```python
from build123d import *

# Parameters (mm, degrees)
SKETCH1_W           = 105
SKETCH1_H           = 105
BOSS_EXTRUDE1_DEPTH = 5
SKETCH2_R           = 5
CUT_EXTRUDE1_DEPTH  = 5
CUT_EXTRUDE2_DEPTH  = 3
FILLET1_R           = 1


with BuildPart() as part:
    # Sketch1 → Boss-Extrude1 (new body)
    with BuildSketch(Plane(origin=(0, 0, 0), x_dir=(1, 0, 0), z_dir=(0, 1, 0))):
        Rectangle(SKETCH1_W, SKETCH1_H)
    extrude(amount=BOSS_EXTRUDE1_DEPTH)

    # Sketch2 → Cut-Extrude1 (cut)
    with BuildSketch(Plane(origin=(0, 5, 0), x_dir=(1, 0, 0), z_dir=(0, 1, 0))):
        with Locations(Location((0, 0, 0), (0, 0, 270))):
            Circle(SKETCH2_R)
    extrude(amount=-CUT_EXTRUDE1_DEPTH, mode=Mode.SUBTRACT)

    # Sketch3 → Cut-Extrude2 (cut)
    with BuildSketch(Plane(origin=(0, 5, 0), x_dir=(1, 0, 0), z_dir=(0, 1, 0))):
        with BuildLine():
            Line((-49.5, -50), (49.5, -50))
            ThreePointArc((49.5, -50), (49.853553391, -49.853553391), (50, -49.5))
            Line((50, -49.5), (50, 49.5))
            ThreePointArc((50, 49.5), (49.853553391, 49.853553391), (49.5, 50))
            Line((49.5, 50), (-49.5, 50))
            ThreePointArc((-49.5, 50), (-49.853553391, 49.853553391), (-50, 49.5))
            Line((-50, 49.5), (-50, -49.5))
            ThreePointArc((-50, -49.5), (-49.853553391, -49.853553391), (-49.5, -50))
        make_face()
    extrude(amount=-CUT_EXTRUDE2_DEPTH, mode=Mode.SUBTRACT)

    # Fillet1
    fillet1_edges = [part.edges().sort_by_distance(p)[0] for p in [
        (52.5, 2.5, 52.5),
        (-52.5, 2.5, 52.5),
        (-52.5, 2.5, -52.5),
        (52.5, 2.5, -52.5),
    ]]
    fillet(fillet1_edges, radius=FILLET1_R)


solid = part.part
```
Input: part model. Units: mm. Frame: model coordinates. A direction names the side the tool comes from. Give positions to 0.01 mm unless a question says otherwise; leave off trailing zeros. Loops run counter-clockwise (first coordinate to the right, second up) from the corner with the lowest first, then second, coordinate; pieces in that order, holes last. Notation, with made-up numbers: M -39.75,-37 L 8.25,-37 A3 ccw 8.25,-32 Z; hole C 29,9.5 d1. An arc over 180 degrees is marked long. Answer as CSV lines item,"result". Start each with the question number.
1. Section C-C on y = 3.35. Return loops of the section in (x, z).
2. Pin query (flat end, axial travel): P1, Ø1.5, axis at x = 17.5, z = -10, coming from the +Y side. Return the tip coordinate at first contact, or that it passes through.
3. Section A-A on z = 0. Return loops of the section in (x, y).
4. Section D-D on z = 45. Return loops of the section in (x, y), plus the area to 3 significant figures.
5. Pull-direction query (X, two-part tool) for faces 3 (the face through (-1, 2, -12)), 4 (the face through (-1, 0, -12)), 5 (the face through (-52.5, 2, 1)); classes: released by +X, released by -X, zero draft, split by the parting line, or undercut.
6. Section B-B on x = 0. Return loops of the section in (y, z).
7. Line query: L1, parallel to X at y = 1.3, z = 0; L2, parallel to X at y = 4.15, z = -12. Output: solid intervals per line, ascending.
8. Reachability of faces 1 (the face through (52.5, 2, 1)), 2 (the face through (1, 4, -50)) from +Z, -Z, +X, -X, +Y, -Y: full face, straight path, thin tool, end or side. Return the list, or none.
Computed values:
1,outline,"M -52.5,-51.5 A1 ccw -51.5,-52.5 L 51.5,-52.5 A1 ccw 52.5,-51.5 L 52.5,51.5 A1 ccw 51.5,52.5 L -51.5,52.5 A1 ccw -52.5,51.5 Z; hole M -50,-49.5 A0.5 ccw -49.5,-50 L 49.5,-50 A0.5 ccw 50,-49.5 L 50,49.5 A0.5 ccw 49.5,50 L -49.5,50 A0.5 ccw -50,49.5 Z"
2,P1,"stops at y = 2"
3,outline,"M -52.5,0 L -5,0 L -5,2 L -50,2 L -50,5 L -52.5,5 Z; M 5,0 L 52.5,0 L 52.5,5 L 50,5 L 50,2 L 5,2 Z"
4,outline,"M -52.5,0 L 52.5,0 L 52.5,5 L 50,5 L 50,2 L -50,2 L -50,5 L -52.5,5 Z"
4,area,"225 mm²"
5,face 3,"undercut"
5,face 4,"zero draft"
5,face 5,"released by -X"
6,outline,"M 0,-52.5 L 5,-52.5 L 5,-50 L 2,-50 L 2,-5 L 0,-5 Z; M 0,5 L 2,5 L 2,50 L 5,50 L 5,52.5 L 0,52.5 Z"
7,L1,"x = -52.5 to -5, 5 to 52.5"
7,L2,"x = -52.5 to -50, 50 to 52.5"
8,face 1,"+Z, -Z, +X, +Y, -Y"
8,face 2,"+Y"
